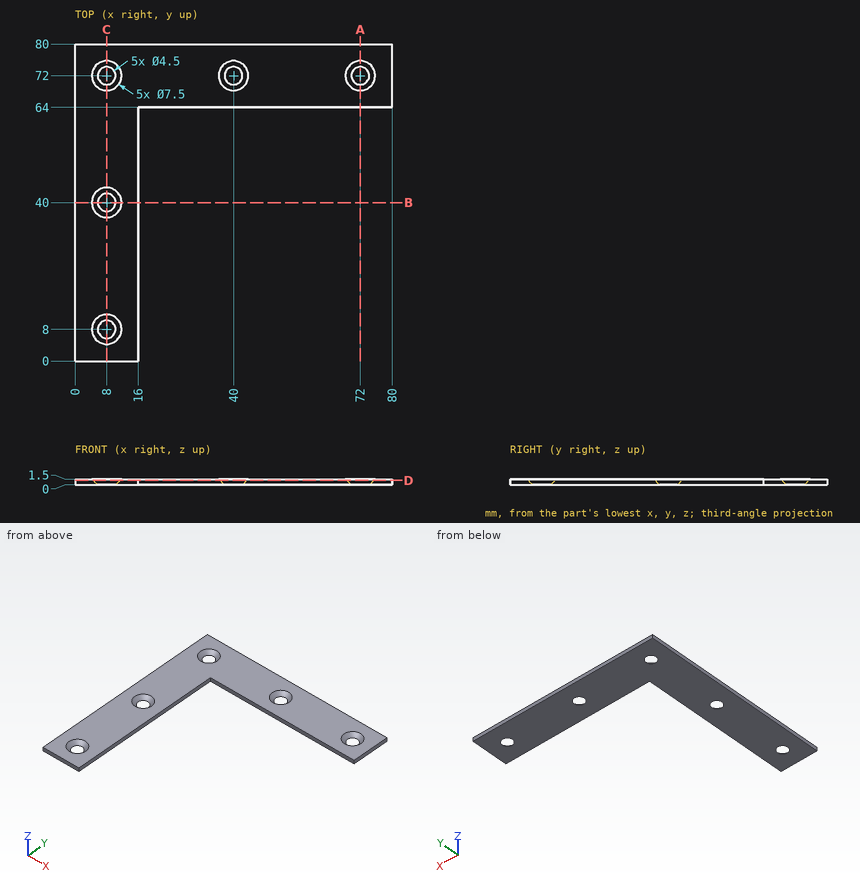
Here's the drawing with two shaded views (mm, measured from the low corner). I have some questions. Round coordinates to 2 decimals unless told otherwise and drop trailing zeros. Loops run counter-clockwise (first coordinate to the right, second up) from the corner with the lowest first, then second, coordinate; pieces in that order, holes last. Notation, with made-up numbers: M 12.5,65.25 L 28.5,65.25 A29 cw 28.5,103.25 Z; hole C 43,47 d10. An arc over 180 degrees is marked long. Answer as a JSON object with one key per item and string values. Group by question number.
Q1. Imagine slicing it at B-B, the plane y = 40. Please give me the cut outline in (x, z).
Q2. Will this pin go through, and if not, where does the flat tip stop? pin 1 (0.8 mm diameter, centred on x = 39.5, z = 1, fed in from -Y).
Q3. Imagine slicing it at D-D, the plane z = 1.15. Please give me the cut outline in (x, y).
Q4. Imagine slicing it at A-A, the plane x = 72. Please give me the cut outline in (y, z), then the cut area to 3 significant figures.
Q5. Please list where these lines run through material, in increasing order: L1, parallel to Y at x = 11, z = 1.3; L2, parallel to Y at x = 6, z = 1.4; L3, parallel to Y at x = 51.5, z = 1.
Q6. Imagine slicing it at C-C, the plane x = 8. Please give me the cut outline in (y, z), then the cut area to 3 significant figures.
Findings:
{
 "1": {"outline": "M 0,0 L 5.75,0 L 4.25,1.5 L 0,1.5 Z; M 10.25,0 L 16,0 L 16,1.5 L 11.75,1.5 Z"},
 "2": {"pin 1": "stops at y = 64"},
 "3": {"outline": "M 0,0 L 16,0 L 16,64 L 80,64 L 80,80 L 0,80 Z; hole C 8,8 d6.8; hole C 8,40 d6.8; hole C 8,72 d6.8; hole C 40,72 d6.8; hole C 72,72 d6.8"},
 "4": {"outline": "M 64,0 L 69.75,0 L 68.25,1.5 L 64,1.5 Z; M 74.25,0 L 80,0 L 80,1.5 L 75.75,1.5 Z", "area": "15.0 mm2"},
 "5": {"L1": "y = 0 to 6.1, 9.9 to 38.1, 41.9 to 70.1, 73.9 to 80", "L2": "y = 0 to 4.95, 11.05 to 36.95, 43.05 to 68.95, 75.05 to 80", "L3": "y = 64 to 80"},
 "6": {"outline": "M 0,0 L 5.75,0 L 4.25,1.5 L 0,1.5 Z; M 10.25,0 L 37.75,0 L 36.25,1.5 L 11.75,1.5 Z; M 42.25,0 L 69.75,0 L 68.25,1.5 L 43.75,1.5 Z; M 74.25,0 L 80,0 L 80,1.5 L 75.75,1.5 Z", "area": "93.0 mm2"}
}
